Source: CAD feature listing. Evaluate the final solid. Frame: model axes, mm. Face numbers are marked on the shaded views. A direction names the side the tool comes from. Coordinates: 2 decimals unless noted, no trailing zeros. Write each loop counter-clockwise with the first axis right and the second up, starting at its lowest first coordinate (ties: lowest second). Pieces come first, ordered by that corner, then holes. Notation, with made-up numbers: M -12.75,58.25 L 40.25,58.25 A17 cw 40.25,72.25 Z; hole C 42,53.25 d4. An arc over 180 degrees is marked long. Write item = value, one per line. Start each with the question number.
1. Section query C-C (y = 88). Output: boundary loops of the cut face in (x, z), then the cut area to 3 significant figures.
2. Line query: line 1 along Y through (x, z) = (15, 44.6); line 2 along X through (y, z) = (50, 43.5); line 3 along X through (y, z) = (20, 38.4). Output: solid intervals per line, ascending.
3. Access query for the marked faces 1, 2 and 3. Directions: +Z, -Z, +X, -X, +Y, -Y. A direction counts if a zero-diameter tool reaches every point of the face in a straight line with its end or side. Return the directions, or none.
4. Pull-direction query (X, two-part tool) for the marked faces 4, 5 and 6; classes: pulls with the +X half, pulls with the -X half, needs draft (parallel to the pull), parting line crosses it, or undercut.
5. Section query B-B (y = 6). Output: boundary loops of the cut face in (x, z), then the cut area to 3 significant figures.
6. Section query A-A (x = -15). Output: boundary loops of the cut face in (y, z).
7. Section query D-D (y = 65). Output: boundary loops of the cut face in (x, z), then the cut area to 4 significant figures.
8. Pin query (flat end, axial travel): pin 1 Ø16 at (x, y) = (32.5, 69.5) entering from -Z; pin 2 Ø22 at (x, y) = (-36.5, 78) entering from -Z; pin 3 Ø1.5 at (x, z) = (9.5, 38.5) entering from -Y; pin 4 Ø4 at (x, z) = (-10, 39.5) entering from +Y. Return the tip coordinate at first contact, or that it passes through.
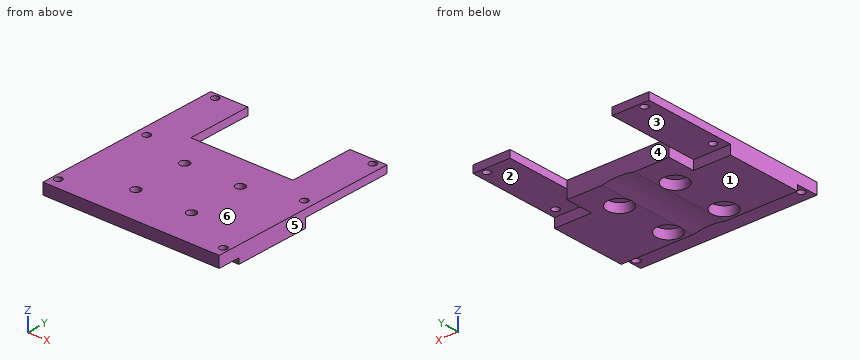
```python
from build123d import *

# Parameters (mm, degrees)
SKETCH1_R                = 37.5
BOSS_EXTRUDE1_DEPTH      = 12
SKETCH2_R                = 30
BOSS_EXTRUDE2_DEPTH      = 56
BOSS_EXTRUDE3_DEPTH      = 5
BOSS_EXTRUDE3_DEPTH_BACK = 1
SKETCH4_W                = 75
SKETCH4_H                = 15
SKETCH4_R                = 3.5
MOVE_FACE3_BY            = 10
MOVE_FACE3_2_BY          = 10
BOSS_EXTRUDE4_DEPTH      = 12
BOSS_EXTRUDE5_DEPTH      = 68
MOVE_FACE1_BY            = 10
SKETCH11_W               = 95
SKETCH11_H               = 15
BOSS_EXTRUDE7_DEPTH      = 20
CUT_EXTRUDE1_DEPTH       = 103.720494547
CUT_EXTRUDE1_DEPTH_BACK  = 103.720494547
SKETCH12_R               = 2.5
SKETCH13_R               = 6.5
CUT_EXTRUDE2_DEPTH       = 5
MOVE_FACE2_BY            = 7
DELETEFACE1_START        = -20
DELETEFACE1_OUTLINE_W    = 95
DELETEFACE1_OUTLINE_H    = 8
DELETEFACE1_DEPTH        = 20
CUT_EXTRUDE3_DEPTH       = 103.359660059
CUT_EXTRUDE3_DEPTH_BACK  = 3
SKETCH15_R               = 2
CUT_EXTRUDE4_DEPTH       = 96.818839484
MOVE_FACE4_BY            = 20
SKETCH16_W               = 55
SKETCH16_H               = 35
CUT_EXTRUDE5_DEPTH       = 10
SKETCH17_W               = 20
SKETCH17_H               = 50
CUT_EXTRUDE6_DEPTH       = 5
SKETCH18_R               = 2
CUT_EXTRUDE7_DEPTH       = 114.535236825


# Read off the part's stored shape, not the designer's step: DeleteFace1
with BuildPart() as part:
    # Sketch1 → Boss-Extrude1 (new body)
    with BuildSketch(Plane(origin=(0, 0, 0), x_dir=(1, 0, 0), z_dir=(0, 1, 0))):
        with Locations(Location((0, 0, 0), (0, 0, 270))):
            Circle(SKETCH1_R)
    extrude(amount=BOSS_EXTRUDE1_DEPTH)

    # Sketch2 → Boss-Extrude2 (add)
    with BuildSketch(Plane(origin=(0, 12, 0), x_dir=(1, 0, 0), z_dir=(0, 1, 0))):
        with Locations(Location((0, 0, 0), (0, 0, 270))):
            Circle(SKETCH2_R)
    extrude(amount=BOSS_EXTRUDE2_DEPTH)


with BuildPart() as body_2:
    # Sketch4 → Boss-Extrude3 (new, two sides: drawn at the far end of the back side and taken through both)
    with BuildSketch(Plane.XY.offset(37.5).offset(-BOSS_EXTRUDE3_DEPTH_BACK)):
        with Locations((0, 75.5)):
            Rectangle(SKETCH4_W, SKETCH4_H)
        with Locations((0, 76)):
            Circle(SKETCH4_R, mode=Mode.SUBTRACT)
    extrude(amount=BOSS_EXTRUDE3_DEPTH + BOSS_EXTRUDE3_DEPTH_BACK)

    # Move Face3: a face moved outward by 10.0
    extrude(body_2.faces().sort_by_distance((-37.5, 75.5, 39.5))[0], amount=MOVE_FACE3_BY, dir=(-1, 0, 0))

    # Move Face3 2: a face moved outward by 10.0
    extrude(body_2.faces().sort_by_distance((37.5, 75.5, 39.5))[0], amount=MOVE_FACE3_2_BY, dir=(1, 0, 0))



with BuildPart() as body_3:
    # Sketch6 → Boss-Extrude4 (new body)
    with BuildSketch(Plane.XZ):
        with BuildLine():
            Line((42.5, 0), (37.5, 0))
            ThreePointArc((37.5, 0), (0, 37.5), (-37.5, 0))
            Line((-37.5, 0), (-42.5, 0))
            ThreePointArc((-42.5, 0), (0, 42.5), (42.5, 0))
        make_face()
    extrude(amount=-BOSS_EXTRUDE4_DEPTH)


with BuildPart() as body_2_1:
    add(body_2.part)

    add(body_3.part)  # Boss-Extrude5 merges body 3
    # Sketch7 → Boss-Extrude5 (add)
    with BuildSketch(Plane.XZ.offset(-68)):
        with BuildLine():
            Line((8.602325267, 36.5), (47.5, 36.5))
            Line((47.5, 36.5), (47.5, 42.5))
            Line((47.5, 42.5), (-47.5, 42.5))
            Line((-47.5, 42.5), (-47.5, 36.5))
            Line((-47.5, 36.5), (-8.602325267, 36.5))
            ThreePointArc((-8.602325267, 36.5), (0, 37.5), (8.602325267, 36.5))
        make_face()
    extrude(amount=BOSS_EXTRUDE5_DEPTH)

    # Move Face1: a face moved outward by 10.0
    extrude(body_2_1.faces().sort_by_distance((0, 41.330789145, 42.5))[0], amount=MOVE_FACE1_BY, dir=(0, 0, 1))

    # Sketch11 → Boss-Extrude7 (add)
    with BuildSketch(Plane.XZ):
        with Locations((0, 45)):
            Rectangle(SKETCH11_W, SKETCH11_H)
    extrude(amount=BOSS_EXTRUDE7_DEPTH)

    # Sketch12 → Cut-Extrude1 (cut, two sides: drawn at the far end of the back side and taken through both)
    with BuildSketch(Plane(origin=(0, 0, 37.5), x_dir=(-1, 0, 0), z_dir=(0, 0, -1)).offset(-CUT_EXTRUDE1_DEPTH_BACK)):
        with Locations((-15, 20)):
            Circle(SKETCH12_R)
        with Locations((15, 20)):
            Circle(SKETCH12_R)
        with Locations((-15, 50)):
            Circle(SKETCH12_R)
        with Locations((15, 50)):
            Circle(SKETCH12_R)
    extrude(amount=CUT_EXTRUDE1_DEPTH + CUT_EXTRUDE1_DEPTH_BACK, mode=Mode.SUBTRACT)

    # Sketch13 → Cut-Extrude2 (cut)
    with BuildSketch(Plane(origin=(0, 0, 36.5), x_dir=(-1, 0, 0), z_dir=(0, 0, -1))):
        with Locations((-15, 50)):
            Circle(SKETCH13_R)
        with Locations((15, 50)):
            Circle(SKETCH13_R)
        with Locations((-15, 20)):
            Circle(SKETCH13_R)
        with Locations((15, 20)):
            Circle(SKETCH13_R)
    extrude(amount=-CUT_EXTRUDE2_DEPTH, mode=Mode.SUBTRACT)

    # Move Face2: a face moved inward by 7.0
    extrude(body_2_1.faces().sort_by_distance((0, 31.294429556, 52.5))[0], amount=MOVE_FACE2_BY, dir=(0, 0, -1), mode=Mode.SUBTRACT)

    # DeleteFace1 outline → DeleteFace1 (cut)
    with BuildSketch(Plane(origin=(0, 0, 0), x_dir=(1, 0, 0), z_dir=(0, 1, 0)).offset(DELETEFACE1_START)):
        with Locations((0, -41.5)):
            Rectangle(DELETEFACE1_OUTLINE_W, DELETEFACE1_OUTLINE_H)
    extrude(amount=DELETEFACE1_DEPTH, mode=Mode.SUBTRACT)

    # Sketch14 → Cut-Extrude3 (cut, two sides: drawn at the far end of the back side and taken through both)
    with BuildSketch(Plane(origin=(0, 0, 36.5), x_dir=(-1, 0, 0), z_dir=(0, 0, -1)).offset(-CUT_EXTRUDE3_DEPTH_BACK)):
        Polygon((47.5, 0), (-42.5, 0), (-47.5, 0), (-47.5, 12), (-42.5, 12), (47.5, 12), align=None)
    extrude(amount=CUT_EXTRUDE3_DEPTH + CUT_EXTRUDE3_DEPTH_BACK, mode=Mode.SUBTRACT)

    # Sketch15 → Cut-Extrude4 (cut, through all)
    with BuildSketch(Plane(origin=(0, 0, 39.5), x_dir=(-1, 0, 0), z_dir=(0, 0, -1))):
        with Locations((44.5, 6)):
            Circle(SKETCH15_R)
        with Locations((-44.5, 6)):
            Circle(SKETCH15_R)
    extrude(amount=-CUT_EXTRUDE4_DEPTH, mode=Mode.SUBTRACT)

    # Move Face4: a face moved outward by 20.0
    extrude(body_2_1.faces().sort_by_distance((0, 83, 41))[0], amount=MOVE_FACE4_BY, dir=(0, 1, 0))

    # Sketch16 → Cut-Extrude5 (cut)
    with BuildSketch(Plane(origin=(0, 0, 36.5), x_dir=(-1, 0, 0), z_dir=(0, 0, -1))):
        with Locations((0, 85.5)):
            Rectangle(SKETCH16_W, SKETCH16_H)
    extrude(amount=-CUT_EXTRUDE5_DEPTH, mode=Mode.SUBTRACT)

    # Sketch17 → Cut-Extrude6 (cut)
    with BuildSketch(Plane(origin=(0, 0, 36.5), x_dir=(-1, 0, 0), z_dir=(0, 0, -1))):
        with Locations((37.5, 78)):
            Rectangle(SKETCH17_W, SKETCH17_H)
        with Locations((-37.5, 78)):
            Rectangle(SKETCH17_W, SKETCH17_H)
    extrude(amount=-CUT_EXTRUDE6_DEPTH, mode=Mode.SUBTRACT)

    # Sketch18 → Cut-Extrude7 (cut, through all)
    with BuildSketch(Plane(origin=(0, 0, 41.5), x_dir=(-1, 0, 0), z_dir=(0, 0, -1))):
        with Locations((-42.5, 58)):
            Circle(SKETCH18_R)
        with Locations((-42.5, 100)):
            Circle(SKETCH18_R)
        with Locations(Location((42.5, 100, 0), (0, 0, 180))):
            Circle(SKETCH18_R)
        with Locations(Location((42.5, 58, 0), (0, 0, 180))):
            Circle(SKETCH18_R)
    extrude(amount=-CUT_EXTRUDE7_DEPTH, mode=Mode.SUBTRACT)


solid = body_2_1.part
```
Results are:
q1.outline = M -47.5,41.5 L -27.5,41.5 L -27.5,45.5 L -47.5,45.5 Z; M 27.5,41.5 L 47.5,41.5 L 47.5,45.5 L 27.5,45.5 Z
q1.area = 160 mm^2
q2.line_1 = 0 to 17.5, 22.5 to 47.5, 52.5 to 68
q2.line_2 = -47.5 to -17.5, -12.5 to 12.5, 17.5 to 47.5
q2.line_3 = -47.5 to -21.5, -8.5 to 8.5, 21.5 to 47.5
q3.face_1 = -Z, +X, -X, +Y, -Y
q3.face_2 = -Z, +X, +Y
q3.face_3 = -Z, -X, +Y
q4.face_4 = undercut
q4.face_5 = pulls with the +X half
q4.face_6 = needs draft
q5.outline = M -47.5,39.5 L -46.5,39.5 L -46.5,45.5 L -47.5,45.5 Z; M -42.5,39.5 L 42.5,39.5 L 42.5,45.5 L -42.5,45.5 Z; M 46.5,39.5 L 47.5,39.5 L 47.5,45.5 L 46.5,45.5 Z
q5.area = 522 mm^2
q6.outline = M 0,39.5 L 12,39.5 L 12,36.5 L 13.5,36.5 L 13.5,41.5 L 17.5,41.5 L 17.5,45.5 L 0,45.5 Z; M 22.5,41.5 L 26.5,41.5 L 26.5,36.5 L 43.5,36.5 L 43.5,41.5 L 47.5,41.5 L 47.5,45.5 L 22.5,45.5 Z; M 52.5,41.5 L 56.5,41.5 L 56.5,36.5 L 68,36.5 L 68,45.5 L 52.5,45.5 Z
q7.outline = M -47.5,41.5 L -27.5,41.5 L -27.5,36.5 L -8.6,36.5 A37.5 cw 8.6,36.5 L 27.5,36.5 L 27.5,41.5 L 47.5,41.5 L 47.5,45.5 L -47.5,45.5 Z
q7.area = 643.5 mm^2
q8.pin_1 = 36.5
q8.pin_2 = 41.5
q8.pin_3 = 12
q8.pin_4 = 68
